Source: CAD feature listing. Evaluate the final solid. Frame: model axes, mm. Face numbers are marked on the shaded views. A direction names the side the tool comes from. Round coordinates to 2 decimals unless told otherwise and drop trailing zeros. Order: outer loops, then holes, each group sorted by start corner. A loop starts at its lowest first (then second) coordinate and runs counter-clockwise, first axis right, second up.
```python
from build123d import *

# Parameters (mm, degrees)
SKETCH1_R           = 1.5
BOSS_EXTRUDE1_DEPTH = 30
SKETCH2_R           = 11
BOSS_EXTRUDE2_DEPTH = 14
SKETCH4_R           = 15
BOSS_EXTRUDE4_DEPTH = 10
BOSS_EXTRUDE4_TAPER = 10
BOSS_EXTRUDE5_START = 3
SKETCH6_R           = 11
BOSS_EXTRUDE5_DEPTH = 3


with BuildPart() as part:
    # Sketch1 → Boss-Extrude1 (new body)
    with BuildSketch(Plane(origin=(0, 0, 0), x_dir=(0, 0, -1), z_dir=(1, 0, 0))):
        Circle(SKETCH1_R)
    boss_extrude1 = extrude(amount=BOSS_EXTRUDE1_DEPTH)

    # Sketch2 → Boss-Extrude2 (add)
    with BuildSketch(Plane(origin=(30, 0, 0), x_dir=(0, 0, -1), z_dir=(1, 0, 0))):
        Circle(SKETCH2_R)
    extrude(amount=BOSS_EXTRUDE2_DEPTH)

    # Sketch4 → Boss-Extrude4 (add)
    with BuildSketch(Plane.ZY.offset(-30)):
        Circle(SKETCH4_R)
    boss_extrude4 = extrude(amount=BOSS_EXTRUDE4_DEPTH, taper=BOSS_EXTRUDE4_TAPER)

    # Mirror2: Boss-Extrude1, Boss-Extrude4 across plane
    add(boss_extrude1.mirror(Plane(origin=(0, 0, 0), x_dir=(0, 0, 1), z_dir=(1, 0, 0))))
    add(boss_extrude4.mirror(Plane(origin=(0, 0, 0), x_dir=(0, 0, 1), z_dir=(1, 0, 0))))

    # Sketch6 → Boss-Extrude5 (add)
    with BuildSketch(Plane.ZY.offset(30).offset(BOSS_EXTRUDE5_START)):
        Circle(SKETCH6_R)
    extrude(amount=-BOSS_EXTRUDE5_DEPTH)


solid = part.part
```
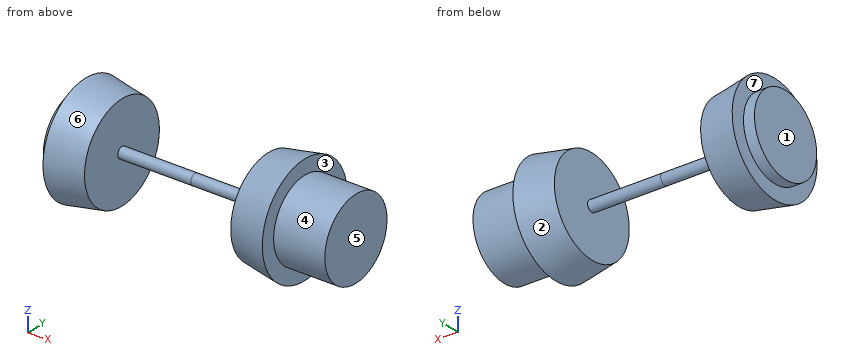
1. Access query for the marked faces 4, 5, 6 and 7. Directions: +Z, -Z, +X, -X, +Y, -Y. A direction counts if a zero-diameter tool reaches every point of the face in a straight line with its end or side. Return the directions, or none.
2. First-contact query: pin 1 (12 mm diameter, centred on x = 5.5, z = -6.5, fed in from +Y). Flat tip, straight axial feed; report the tip coordinate or a pass-through.
3. Section B-B on x = 18. Return loops of the section in (y, z).
4. Section A-A on z = 0. Return loops of the section in (x, y).
5. Line query: line 1 along X through (y, z) = (5, -7.5); line 2 along X through (y, z) = (-10, -8); line 3 along Z through (x, y) = (33.5, -8). Output: solid intervals per line, ascending.
6. Pull-direction query (X, two-part tool) for the marked faces 1, 2 and 3; classes: released by +X, released by -X, zero draft, split by the parting line, or undercut.
Result:
1. face 4: +X
1. face 5: +Z, -Z, +X, +Y, -Y
1. face 6: none
1. face 7: -X
2. pin 1: stops at y = 1.41
3. outline: circle Ø3 at (0, 0)
4. outline: (-33, -11) - (-30, -11) - (-30, -15) - (-20, -13.24) - (-20, -1.5) - (20, -1.5) - (20, -13.24) - (30, -15) - (30, -11) - (44, -11) - (44, 11) - (30, 11) - (30, 15) - (20, 13.24) - (20, 1.5) - (-20, 1.5) - (-20, 13.24) - (-30, 15) - (-30, 11) - (-33, 11) - close
5. line 1: x = -33 to -20, 20 to 44
5. line 2: x = -30 to -20, 20 to 30
5. line 3: z = -7.55 to 7.55
6. face 1: released by -X
6. face 2: undercut
6. face 3: released by +X
